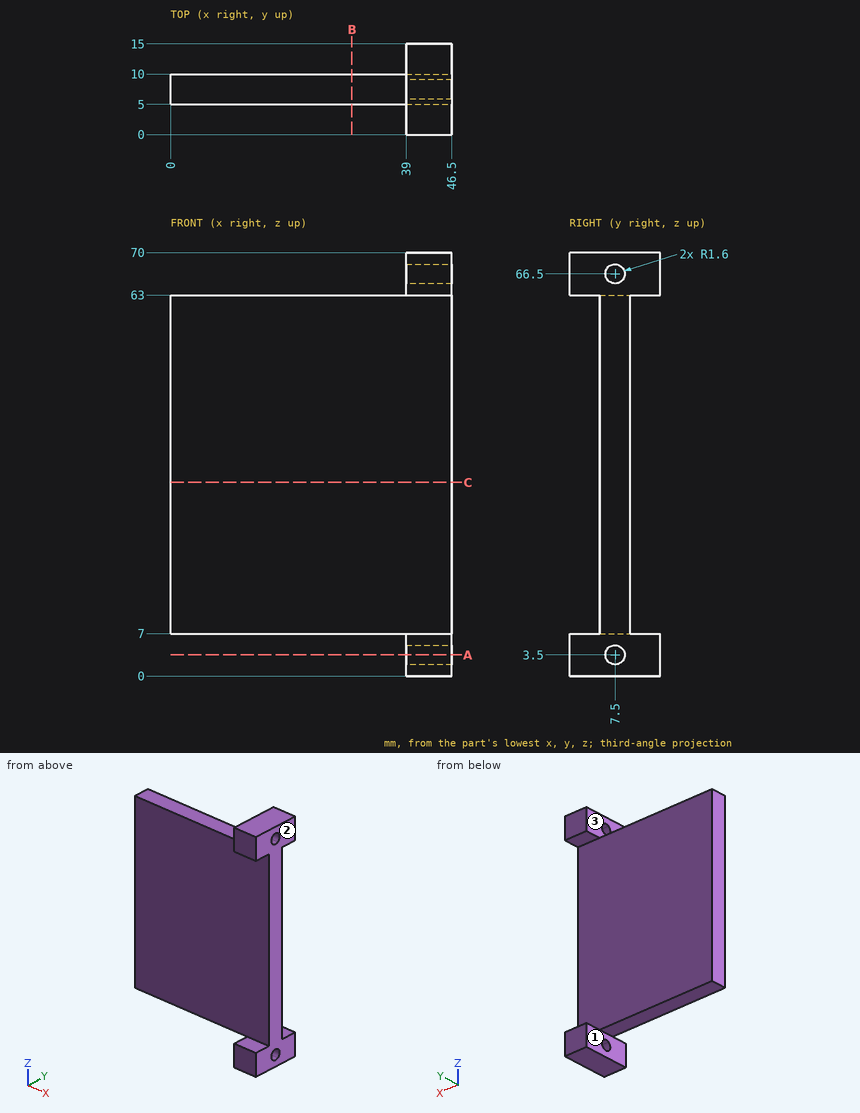
Verification items for this drawing (mm, ordinates from the low corner). A direction names the side the tool comes from. Round coordinates to 2 decimals unless told otherwise and drop trailing zeros. Loops run counter-clockwise (first coordinate to the right, second up) from the corner with the lowest first, then second, coordinate; pieces in that order, holes last. Notation, with made-up numbers: (-38, -33.75) -> (18, -33.75) arc R12 ccw to (18, -16.75) -> close; hole circle Ø11 at (33.25, 75). An arc over 180 degrees is marked (long way). Write item = value, one per line. Start each with the question number.
1) Sectioned sample at A-A, the plane z = 3.5. Record the cut outline in (x, y).
2) Sectioned sample at C-C, the plane z = 32. Record the cut outline in (x, y).
3) Gauge pin test, flat ends, axial feed: pin 1 Ø6 at (y, z) = (2.5, 28.5) entering from -X; pin 2 Ø6 at (x, y) = (35.5, 8.5) entering from +Z; pin 3 Ø23 at (x, z) = (15, 24) entering from -Y; pin 4 Ø3.5 at (y, z) = (10, 67) entering from -X. Record the tip position at first contact, or that the pin passes through.
4) Sectioned sample at B-B, the plane x = 30. Record the cut outline in (y, z), plus the area to 3 significant figures.
5) Thickness scan on probe 1 along Z at (x, y) = (40, 13); probe 2 along Z at (x, y) = (25.5, 7.75); probe 3 along Y at (x, z) = (40, 52.5). Record the ranges inside material, lowest first.
6) Set-up check for the marked faces 1, 2 and 3: record each of +Z, -Z, +X, -X, +Y, -Y from which the full face is reachable in a straight line by a thin tool's end or side.
Results are:
q1.outline = (39, 0) -> (46.5, 0) -> (46.5, 5.9) -> (39, 5.9) -> close; (39, 9.1) -> (46.5, 9.1) -> (46.5, 15) -> (39, 15) -> close
q2.outline = (0, 5) -> (46.5, 5) -> (46.5, 10) -> (0, 10) -> close
q3.pin_1 = 0
q3.pin_2 = 63
q3.pin_3 = 5
q3.pin_4 = 39
q4.outline = (5, 7) -> (10, 7) -> (10, 63) -> (5, 63) -> close
q4.area = 280 mm^2
q5.probe_1 = 0 to 7, 63 to 70
q5.probe_2 = 7 to 63
q5.probe_3 = 5 to 10
q6.face_1 = -Z, -X, +Y, -Y
q6.face_2 = +Z, -Z, +X, +Y, -Y
q6.face_3 = +Z, -X, +Y, -Y
